Can you work these out from the model? Positions are in its coordinate system, mm. A direction names the side the tool comes from. Coordinates: 2 decimals unless noted, no trailing zeros. Order: outer loops, then holes, each group sorted by start corner. A loop starts at its lowest first (then second) coordinate and runs counter-clockwise, first axis right, second up. Notation, with made-up numbers: (46.25, 35) -> (104.25, 35) arc R17 cw to (104.25, 43) -> close; hole circle Ø6 at (-15, 33). An arc over 180 degrees is marked (long way). Answer in a Markdown table with one row per item. Add a question column.
1. Imagine slicing it at A-A on z = 7.5. Write out the boundary of the cut face in (x, y).
2. Imagine slicing it at C-C on x = -62.5. Write out the boundary of the cut face in (y, z), plus the area to 3 significant figures.
3. If I drill on line 1 along X through (y, z) = (5.25, 43.75); line 2 along X through (y, z) = (3.75, 7.5); line 3 along Z through (x, y) = (64.5, 7), over which ranges is the centre line in solid material (lowest first)? Write a range as [from, to].
4. Imagine slicing it at B-B on y = 5.25. State how many separate pieces and enclosed holes the cut face has, plus the area to 3 significant figures.
5. On a 3-axis mill with a long thin cutter (end or side, diameter ignored), from which of +Z, -Z, +X, -X, +Y, -Y can I reach the whole of each face in a straight line? I mean faces 4 (the face through (-6.35, 1.52, -24.49)), 5 (the face through (1, 10, 1)). Say none if no direction works.
6. Will these pins go through, and if not, where does the flat tip stop? pin 1 (13 mm diameter, centred on x = -8, z = 46, fed in from -Y); pin 2 (4.5 mm diameter, centred on x = -62.5, z = -62.5, fed in from +Y); pin 3 (3.5 mm diameter, centred on x = 9.5, z = 45, fed in from -Y).
7. We'd pull the mould along X, two halves only. Please class faces 1 (the face through (-70.15, 5.07, 69.89)), 2 (the face through (1, 0, 1)), 3 (the face through (11, 3, -32)): pulls with the +X half, pulls with the -X half, needs draft (parallel to the pull), parting line crosses it, or undercut.
Autodesk Inventor part; units mm, degrees
ref_plane "YZ Plane" through (0, 0, 0) normal (1, 0, 0) x (0, 1, 0)
ref_plane "XZ Plane" through (0, 0, 0) normal (0, 1, 0) x (-1, 0, 0)
ref_plane "XY Plane" through (0, 0, 0) normal (0, 0, 1) x (1, 0, 0)
sketch "Sketch1" plane through (0, 0, 0) normal (0, 1, 0) x (-1, 0, 0)
  line L0 (75, 75) -> (-75, 75)
  line L1 (-75, 75) -> (-75, -75)
  line L2 (-75, -75) -> (75, -75)
  line L3 (75, -75) -> (75, 75)
  line L4 (75, 75) -> (-75, -75) construction
  line L5 (-75, 75) -> (75, -75) construction
  point P0 (0, 0)
  dimension "d0" = 150
  dimension "d1" = 150
extrude "Extrusion1" add sketch "Sketch1" along normal blind 10
sketch "Sketch2" plane through (0, 10, 0) normal (0, 1, 0) x (1, 0, 0)
  line L0 (-10, 43.75) -> (10, 43.75)
  line L1 (10, 43.75) -> (10, -43.75)
  line L2 (10, -43.75) -> (-10, -43.75)
  line L3 (-10, -43.75) -> (-10, 43.75)
  line L4 (-10, -29.25) -> (10, -29.25)
  line L5 (10, -29.25) -> (10, 29.25)
  line L6 (10, 29.25) -> (-10, 29.25)
  line L7 (-10, 29.25) -> (-10, -29.25)
  circle A0 centre (-10, 43.75) radius 2.5
  circle A1 centre (10, 43.75) radius 2.5
  circle A2 centre (-10, 29.25) radius 2.5
  circle A3 centre (10, 29.25) radius 2.5
  circle A4 centre (10, -29.25) radius 2.5
  circle A5 centre (-10, -29.25) radius 2.5
  circle A6 centre (-10, -43.75) radius 2.5
  circle A7 centre (10, -43.75) radius 2.5
  line L8 (-75, 75) -> (-75, -75)
  point P0 (0, 0)
  dimension "d4" = 20
  dimension "d5" = 87.5
  dimension "d6" = 58.5
  dimension "d7" = 5
  dimension "d8" = 5
  dimension "d9" = 5
  dimension "d10" = 5
  dimension "d11" = 5
  dimension "d12" = 5
  dimension "d13" = 5
  dimension "d14" = 5
  dimension "d51" = 75
extrude "Extrusion2" cut sketch "Sketch2" against normal through all contours L3 A0 L0 | L0 A0 L3 | A1 L1 L0 | L0 L1 A1 | A2 L6 L3 | L3 A2 | L6 A2 L3 | A3 L1 | L1 L6 A3 | L6 L1 A3 | A5 L4 L3 | L3 A5 | L4 A5 L3 | A4 L1 | L1 L4 A4 | L4 L1 A4 | A6 L2 L3 | L3 L2 A6 | A7 L2 L1 | L1 L2 A7
fillet "Fillet1" radius 17 4 edges at (75, 5, 75) (-75, 5, 75) (75, 5, -75) (-75, 5, -75)
sketch "Sketch5" plane through (0, 0, 0) normal (0, -1, 0) x (1, 0, 0)
  circle A0 centre (-10, 43.75) radius 2.5
  circle A1 centre (10, 43.75) radius 2.5
  circle A2 centre (-10, 29.25) radius 2.5
  circle A3 centre (10, 29.25) radius 2.5
  circle A4 centre (-10, -29.25) radius 2.5
  circle A5 centre (10, -29.25) radius 2.5
  circle A6 centre (-10, -43.75) radius 2.5
  circle A7 centre (10, -43.75) radius 2.5
  point P0 (0, 0)
hole "Hole2" at (-10, 0, 43.75) at (10, 0, 43.75) at (-10, 0, 29.25) at (10, 0, 29.25) at (-10, 0, -29.25) at (10, 0, -29.25) at (-10, 0, -43.75) at (10, 0, -43.75) direction (0, 1, 0) diameter 5.5 end through all counterbore diameter 12 counterbore depth 3
sketch "Sketch6" plane through (0, 10, 0) normal (0, 1, 0) x (1, 0, 0)
  line L0 (62.5, 62.5) -> (-62.5, 62.5) construction
  line L1 (-62.5, 62.5) -> (-62.5, -62.5) construction
  line L2 (-62.5, -62.5) -> (62.5, -62.5) construction
  line L3 (62.5, -62.5) -> (62.5, 62.5) construction
  line L4 (62.5, 62.5) -> (-62.5, -62.5) construction
  line L5 (-62.5, 62.5) -> (62.5, -62.5) construction
  point P0 (0, 0)
  dimension "d80" = 125
  dimension "d81" = 125
hole "Hole3" at (62.5, 10, -62.5) at (62.5, 10, 62.5) at (-62.5, 10, -62.5) at (-62.5, 10, 62.5) direction (0, -1, 0) diameter 5.2 end through all
sketch "Sketch7" plane through (0, 10, 0) normal (0, 1, 0) x (1, 0, 0)
  line L0 (7.5, -7.5) -> (-7.5, -7.5) construction
  line L1 (-7.5, -7.5) -> (-7.5, 7.5) construction
  line L2 (-7.5, 7.5) -> (7.5, 7.5) construction
  line L3 (7.5, 7.5) -> (7.5, -7.5) construction
  line L4 (7.5, -7.5) -> (-7.5, 7.5) construction
  line L5 (-7.5, -7.5) -> (7.5, 7.5) construction
  circle A0 centre (7.5, -7.5) radius 2.75
  circle A1 centre (-7.5, -7.5) radius 2.75
  circle A2 centre (7.5, 7.5) radius 2.75
  circle A3 centre (-7.5, 7.5) radius 2.75
  point P0 (0, 0)
  dimension "d89" = 15
  dimension "d90" = 15
  dimension "d91" = 5.5
  dimension "d92" = 5.5
  dimension "d93" = 5.5
  dimension "d94" = 5.5
extrude "Extrusion4" cut sketch "Sketch7" against normal through all
equation "\"d91\" = d94"
equation "\"d92\" = d94"
equation "\"d93\" = d94"
properties part number "VerticalActuationMount" material "ABS Plastic"
Answers follow:
| question | item | result |
|---|---|---|
| 1 | outline | (-75, 0) -> (-10.25, 0) -> (-10.25, 10) -> (-75, 10) -> close; (-4.75, 0) -> (4.75, 0) -> (4.75, 10) -> (-4.75, 10) -> close; (10.25, 0) -> (75, 0) -> (75, 10) -> (10.25, 10) -> close |
| 2 | outline | (0, -74.39) -> (10, -74.39) -> (10, -65.1) -> (0, -65.1) -> close; (0, -59.9) -> (10, -59.9) -> (10, 59.9) -> (0, 59.9) -> close; (0, 65.1) -> (10, 65.1) -> (10, 74.39) -> (0, 74.39) -> close |
| 2 | area | 1,380 mm² |
| 3 | line 1 | x = [-75, -12.75], [-7.25, 7.25], [12.75, 75] |
| 3 | line 2 | x = [-75, -10.25], [-4.75, 4.75], [10.25, 75] |
| 3 | line 3 | z = [-73.71, -64.16], [-60.84, 60.84], [64.16, 73.71] |
| 4 | separate pieces | 1 |
| 4 | enclosed holes | 16 |
| 4 | area | 21,900 mm² |
| 5 | face 4 | -Y |
| 5 | face 5 | +Z, -Z, +X, -X, +Y |
| 6 | pin 1 | stops at y = 0 |
| 6 | pin 2 | passes through |
| 6 | pin 3 | stops at y = 3 |
| 7 | face 1 | pulls with the -X half |
| 7 | face 2 | needs draft |
| 7 | face 3 | undercut |
